```python
from build123d import *

# Parameters (mm, degrees)
SKETCH_1_W             = 459
SKETCH_1_H             = 50
SM_BASE_FLANGE_1_DEPTH = 8
OTHER_START            = -25
OTHER_1_DEPTH          = 50
OTHER_1_2_DEPTH        = 50
CHAMFER_1_SIZE         = 10
CUT_EXTRUDE_1_DEPTH    = 461.532300713
M8X1_251_D             = 6.8
M8X1_251_CSINK_D       = 8.5
M8X1_251_CSINK_ANGLE   = 90


# Read off the part's stored shape, not the designer's step: Изгиб1
# Sheet-metal steps are written as plain solids
with BuildPart() as part:
    # Sketch 1 → Базовая кромка1 (new body)
    with BuildSketch(Plane(origin=(0, 0, 0), x_dir=(1, 0, 0), z_dir=(0, 1, 0))):
        with Locations((-229.5, 0)):
            Rectangle(SKETCH_1_W, SKETCH_1_H)
    extrude(amount=SM_BASE_FLANGE_1_DEPTH)

    # Other 1 outline → Other 1 (cut)
    with BuildSketch(Plane.XY.offset(OTHER_START)):
        with BuildLine():
            Line((-392.872583002, 8), (-396.186291703, 4.686291703))
            ThreePointArc((-396.186291703, 4.686291703), (-401.377065191, 1.217927743), (-407.5, 2.85e-07))
            Line((-407.5, 2.85e-07), (0, 0))
            Line((0, 0), (0, 8))
            Line((0, 8), (-392.872583002, 8))
        make_face()
    extrude(amount=OTHER_1_DEPTH, mode=Mode.SUBTRACT)

    # Other 1 2 outline → Other 1 2 (add)
    with BuildSketch(Plane.XY.offset(OTHER_START)):
        with BuildLine():
            Line((-407.5, 8.000000285), (-392.872583002, 8))
            Line((-392.872583002, 8), (-375.21572863, 25.656854127))
            ThreePointArc((-375.21572863, 25.656854127), (-372.620341896, 27.3910361), (-369.558874503, 27.999999827))
            Line((-369.558874503, 27.999999827), (0, 28))
            Line((0, 28), (0, 36))
            Line((0, 36), (-369.558874503, 35.999999827))
            ThreePointArc((-369.558874503, 35.999999827), (-375.681809355, 34.78207236), (-380.87258288, 31.313708377))
            Line((-380.87258288, 31.313708377), (-401.843145952, 10.343145952))
            ThreePointArc((-401.843145952, 10.343145952), (-404.43853265, 8.608964003), (-407.5, 8.000000285))
        make_face()
    extrude(amount=OTHER_1_2_DEPTH)

    # Фаска1
    chamfer_1_edges = [part.edges().sort_by_distance(p)[0] for p in [
        (-459, 4, -25),
        (-459, 4, 25),
    ]]
    chamfer(chamfer_1_edges, length=CHAMFER_1_SIZE)

    # Эскиз4 → Вытянуть1 (cut, through all)
    with BuildSketch(Plane(origin=(0, 8, 0), x_dir=(1, 0, 0), z_dir=(0, 1, 0))):
        with BuildLine():
            Line((-435, 8.5), (-459, 8.5))
            Line((-459, 8.5), (-459, -8.5))
            Line((-459, -8.5), (-435, -8.5))
            ThreePointArc((-435, -8.5), (-426.5, 0), (-435, 8.5))
        make_face()
    extrude(amount=-CUT_EXTRUDE_1_DEPTH, mode=Mode.SUBTRACT)

    # Зеркальное отражение1: part across plane


with BuildPart() as part_1:
    add(part.part)
    add(part.part.mirror(Plane(origin=(0, 36, -25), x_dir=(0, 0, 1), z_dir=(-1, 0, 0))))

    # Отверстие обработанное метчиком M8x1.251 (through all)
    with Locations(Plane.XZ.offset(-28)):
        with Locations((-325, -1.5), (-300, -1.5), (-300, -17.5), (-325, -17.5), (300, -1.5), (325, -1.5), (325, -17.5), (300, -17.5), (-255.5, 8), (-239.5, -8), (-239.5, 8), (239.5, 8), (239.5, -8), (255.5, 8)):
            CounterSinkHole(M8X1_251_D / 2, M8X1_251_CSINK_D / 2, counter_sink_angle=M8X1_251_CSINK_ANGLE)


solid = part_1.part
```
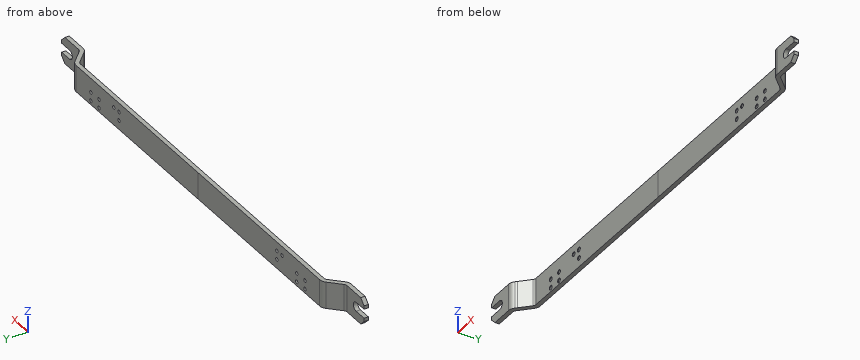
Geometry check sheet. Reference: the model listing, model coordinates, mm. Coordinates: 2 decimals unless noted, no trailing zeros. Write each loop counter-clockwise with the first axis right and the second up, starting at its lowest first coordinate (ties: lowest second). Pieces come first, ordered by that corner, then holes. Notation, with made-up numbers: (59, 12) -> (93, 12) arc R34 cw to (93, 45) -> close; hole circle Ø2 at (29.25, -3). An arc over 180 degrees is marked (long way). Use CSV: the item, a comma, the result in double quotes. Start each with the question number.
Item 1: Cross-section at B-B, the plane x = 283.5. Record the cut outline in (y, z), plus the area to 3 significant figures.
Item 2: Thickness scan on line 1 (Z direction, x = 300, y = 31); line 2 (Z direction, x = 239, y = 30); line 3 (X direction, y = 31, z = 8). Record the ranges inside material, lowest first.
Item 3: Cross-section at A-A, the plane y = 20. Record the cut outline in (x, z).
Item 4: Depth check by flat-ended pin: pin 1 Ø11 at (x, z) = (-325, -1.5) entering from +Y; pin 2 Ø11 at (x, z) = (-239.5, 8) entering from -Y; pin 3 Ø15 at (x, z) = (-425, 8.5) entering from +Y; pin 4 Ø8 at (y, z) = (28.5, -11.5) entering from +X. Enter the tip coordinate at first touch or a pass-through.
Answers:
1,outline,"(28, -25) -> (36, -25) -> (36, 25) -> (28, 25) -> close"
1,area,"400 mm^2"
2,line 1,"-25 to -20.9, -14.1 to -4.9, 1.9 to 25"
2,line 2,"-25 to -11.36, -4.64 to 4.64, 11.36 to 25"
2,line 3,"-381.19 to -258.9, -252.1 to -242.9, -236.1 to 236.1, 242.9 to 252.1, 258.9 to 381.19"
3,outline,"(-392.19, -25) -> (-380.87, -25) -> (-380.87, 25) -> (-392.19, 25) -> close; (380.87, -25) -> (392.19, -25) -> (392.19, 25) -> (380.87, 25) -> close"
4,pin 1,"y = 36"
4,pin 2,"y = 28"
4,pin 3,"y = 8"
4,pin 4,"x = 387.69"
